```python
from build123d import *

# Parameters (mm, degrees)
BOSS_EXTRUDE1_DEPTH  = 330.2
REVOLVE1_ANGLE       = 90
MIRROR2_COPY_1_DEPTH = 330.2
MIRROR2_COPY_2_ANGLE = 90


with BuildPart() as part:
    # Sketch1 → Boss-Extrude1 (new body)
    with BuildSketch(Plane.XY):
        with BuildLine():
            Line((0, 12.7), (177.8, 12.7))
            ThreePointArc((177.8, 12.7), (204.740768363, 23.859231637), (215.9, 50.8))
            Line((215.9, 50.8), (215.9, 381))
            ThreePointArc((215.9, 381), (182.42230509, 461.82230509), (101.6, 495.3))
            Line((101.6, 495.3), (0, 495.3))
            Line((0, 495.3), (0, 508))
            Line((0, 508), (101.6, 508))
            ThreePointArc((101.6, 508), (191.402561211, 470.802561211), (228.6, 381))
            Line((228.6, 381), (228.6, 50.8))
            ThreePointArc((228.6, 50.8), (213.721024484, 14.878975516), (177.8, 0))
            Line((177.8, 0), (0, 0))
            Line((0, 0), (0, 12.7))
        make_face()
    boss_extrude1 = extrude(amount=BOSS_EXTRUDE1_DEPTH)

    # Sketch1<2> → Revolve1 (revolve)
    with BuildSketch(Plane.XY):
        with BuildLine():
            Line((0, 12.7), (177.8, 12.7))
            ThreePointArc((177.8, 12.7), (204.740768363, 23.859231637), (215.9, 50.8))
            Line((215.9, 50.8), (215.9, 381))
            ThreePointArc((215.9, 381), (182.42230509, 461.82230509), (101.6, 495.3))
            Line((101.6, 495.3), (0, 495.3))
            Line((0, 495.3), (0, 508))
            Line((0, 508), (101.6, 508))
            ThreePointArc((101.6, 508), (191.402561211, 470.802561211), (228.6, 381))
            Line((228.6, 381), (228.6, 50.8))
            ThreePointArc((228.6, 50.8), (213.721024484, 14.878975516), (177.8, 0))
            Line((177.8, 0), (0, 0))
            Line((0, 0), (0, 12.7))
        make_face()
    revolve1 = revolve(axis=Axis((0, 0, 0), (0, 1, 0)), revolution_arc=REVOLVE1_ANGLE)

    # Mirror1: Boss-Extrude1, Revolve1 across plane
    add(boss_extrude1.mirror(Plane(origin=(0, 0, 0), x_dir=(0, 0, 1), z_dir=(1, 0, 0))))
    add(revolve1.mirror(Plane(origin=(0, 0, 0), x_dir=(0, 0, 1), z_dir=(1, 0, 0))))

    # Mirror2: Boss-Extrude1, Revolve1 across plane
    add(boss_extrude1.mirror(Plane(origin=(177.8, 50.8, 330.2), x_dir=(1, 0, 0), z_dir=(0, 0, 1))))
    add(revolve1.mirror(Plane(origin=(177.8, 50.8, 330.2), x_dir=(1, 0, 0), z_dir=(0, 0, 1))))

    # Mirror2 copy 1 sketch → Mirror2 copy 1 (add)
    with BuildSketch(Plane(origin=(0, 0, 660.4), x_dir=(-1, 0, 0), z_dir=(0, 0, -1))):
        with BuildLine():
            Line((0, 12.7), (177.8, 12.7))
            ThreePointArc((177.8, 12.7), (204.740768363, 23.859231637), (215.9, 50.8))
            Line((215.9, 50.8), (215.9, 381))
            ThreePointArc((215.9, 381), (182.42230509, 461.82230509), (101.6, 495.3))
            Line((101.6, 495.3), (0, 495.3))
            Line((0, 495.3), (0, 508))
            Line((0, 508), (101.6, 508))
            ThreePointArc((101.6, 508), (191.402561211, 470.802561211), (228.6, 381))
            Line((228.6, 381), (228.6, 50.8))
            ThreePointArc((228.6, 50.8), (213.721024484, 14.878975516), (177.8, 0))
            Line((177.8, 0), (0, 0))
            Line((0, 0), (0, 12.7))
        make_face()
    extrude(amount=MIRROR2_COPY_1_DEPTH)

    # Mirror2 copy 2 sketch → Mirror2 copy 2 (revolve)
    with BuildSketch(Plane(origin=(0, 0, 660.4), x_dir=(-1, 0, 0), z_dir=(0, 0, -1))):
        with BuildLine():
            Line((0, 12.7), (177.8, 12.7))
            ThreePointArc((177.8, 12.7), (204.740768363, 23.859231637), (215.9, 50.8))
            Line((215.9, 50.8), (215.9, 381))
            ThreePointArc((215.9, 381), (182.42230509, 461.82230509), (101.6, 495.3))
            Line((101.6, 495.3), (0, 495.3))
            Line((0, 495.3), (0, 508))
            Line((0, 508), (101.6, 508))
            ThreePointArc((101.6, 508), (191.402561211, 470.802561211), (228.6, 381))
            Line((228.6, 381), (228.6, 50.8))
            ThreePointArc((228.6, 50.8), (213.721024484, 14.878975516), (177.8, 0))
            Line((177.8, 0), (0, 0))
            Line((0, 0), (0, 12.7))
        make_face()
    revolve(axis=Axis((0, 0, 660.4), (0, 1, 0)), revolution_arc=MIRROR2_COPY_2_ANGLE)


solid = part.part
```
Verification items for the finished model (mm, model axes). A direction names the side the tool comes from. Round coordinates to 2 decimals unless told otherwise and drop trailing zeros. Write each loop counter-clockwise with the first axis right and the second up, starting at its lowest first coordinate (ties: lowest second). Pieces come first, ordered by that corner, then holes.
1. Gauge pin test, flat ends, axial feed: P1, Ø10, axis at x = 141, y = 192, coming from the +Z side; P2, Ø6, axis at x = -118.5, y = 298, coming from the +Z side; P3, Ø2, axis at y = 387.5, z = 337, coming from the +X side. Record the tip position at first contact, or that the pin passes through.
2. Draft check along Z on faces 3 (the cylindrical face through (-214.114, 15.276, 334.823)), 4 (the cylindrical face through (-5.027, 213.589, 888.945)), 5 (the cylindrical face through (-204.44, 23.56, 334.82)). Enter one of: +Z half, -Z half, draft (parallel to the pull), parting line (faces both ways), or undercut.
3. Access from +Z, -Z, +X, -X, +Y, -Y to the whole of each face (thin tool, end or side, straight path). Record for faces 1 (the flat face through (-1, 508, 336)), 2 (the flat face through (215.9, 214, 335)).
4. Section check B-B on y = 332.5. Enter the section's corners in (x, z).
5. Scan lines: L1, parallel to X at y = 145, z = 463; L2, parallel to Y at x = -30, z = 71; L3, parallel to X at y = 44, z = 62. Record each from-to range of solid material in increasing order.
6. Section check A-A on z = 625.5. Enter the section's corners in (x, y).
Answer:
1. P1: stops at z = 844.14
1. P2: stops at z = 857.68
1. P3: stops at x = 228.48
2. face 3: draft
2. face 4: +Z half
2. face 5: undercut
3. face 1: +Z, -Z, +X, -X, +Y
3. face 2: none
4. outline: (-228.6, 0) arc R228.6 ccw to (228.6, 0) - (228.6, 660.4) arc R228.6 ccw to (-228.6, 660.4) - close; hole (-215.9, 0) arc R215.9 ccw to (215.9, 0) - (215.9, 660.4) arc R215.9 ccw to (-215.9, 660.4) - close
5. L1: x = -228.6 to -215.9, 215.9 to 228.6
5. L2: y = 0 to 12.7, 495.3 to 508
5. L3: x = -228.14 to -215.29, 215.29 to 228.14
6. outline: (-228.6, 50.8) arc R50.8 ccw to (-177.8, 0) - (177.8, 0) arc R50.8 ccw to (228.6, 50.8) - (228.6, 381) arc R127 ccw to (101.6, 508) - (-101.6, 508) arc R127 ccw to (-228.6, 381) - close; hole (-215.9, 50.8) arc R38.1 ccw to (-177.8, 12.7) - (177.8, 12.7) arc R38.1 ccw to (215.9, 50.8) - (215.9, 381) arc R114.3 ccw to (101.6, 495.3) - (-101.6, 495.3) arc R114.3 ccw to (-215.9, 381) - close
